Geometry: final body of the model. Coordinates: model frame, mm. A direction names the side the tool comes from. Coordinates: 2 decimals unless noted, no trailing zeros. Order: outer loops, then holes, each group sorted by start corner. A loop starts at its lowest first (then second) coordinate and runs counter-clockwise, first axis right, second up. Notation, with made-up numbers: M 12.5,32.25 L 46.5,32.25 A17 cw 46.5,62.25 Z; hole C -7,12 d4. An arc over 180 degrees is marked long. Write item = value, one per line. Start each with the question number.
```python
from build123d import *

# Parameters (mm, degrees)
F0_W     = 92.1045392752
F0_H     = 59.6973858774
F1_DEPTH = 25.4
F2_DEPTH = 25.4
F4_W     = 34.4229061157
F4_H     = 23.5688388348
F5_DEPTH = 70.612
F6_DEPTH = 99.568


with BuildPart() as f1:
    # F0 (on Front) → F1 (new body)
    with BuildSketch(Plane.XZ):
        with Locations((-26.6700014472, 29.8486929387)):
            Rectangle(F0_W, F0_H)
    extrude(amount=F1_DEPTH)

    # F2 (add): a face of the model
    f2_faces = [f1.faces().sort_by_distance(p)[0] for p in [
        (-26.6700014472, 0, 29.8486929387),
    ]]
    extrude(f2_faces, amount=F2_DEPTH)

    # F4 (on face) → F5 (cut)
    with BuildSketch(Plane.XZ.offset(25.4)):
        with Locations((-26.9801160321, 47.91296646)):
            Rectangle(F4_W, F4_H)
    extrude(amount=-F5_DEPTH, mode=Mode.SUBTRACT)

    # F3 (on face) → F6 (cut)
    with BuildSketch(Plane.YZ.offset(19.3822681904)):
        with BuildLine():
            Line((-25.4, 59.6973858774), (-25.4, 12.8698255867))
            ThreePointArc((-25.4, 12.8698255867), (1.6694190997, 29.9515872227), (13.4900575504, 59.6973858774))
            Line((13.4900575504, 59.6973858774), (-25.4, 59.6973858774))
        make_face()
    extrude(amount=-F6_DEPTH, mode=Mode.SUBTRACT)


solid = f1.part
```
Item 1: First-contact query: pin 1 (1.5 mm diameter, centred on x = -52, z = 28, fed in from -Y); pin 2 (6 mm diameter, centred on x = -24, y = 20, fed in from +Z). Flat tips, straight axial feed; report the tip coordinate or a pass-through.
Item 2: Material intervals for probe 1 along X at (y, z) = (18.5, 55.5); probe 2 along Y at (x, z) = (-64, 16); probe 3 along Z at (x, y) = (-11.5, 19), sorted ascending. Write a range as [from, to].
Item 3: Draft query along X for faces 1 (the flat face through (-9.769, 18, 48)), 2 (the flat face through (-44.192, 18, 48)), 3 (the flat face through (-72.722, 5, 23)), 4 (the flat face through (5, 19, 59.697)). Return one class per face: pulls with the +X half, pulls with the -X half, needs draft (parallel to the pull), parting line crosses it, or undercut.
Item 4: Section query A-A on y = 15. Output: boundary loops of the cut face in (x, z).
Item 5: Section query C-C on x = -5. Output: boundary loops of the cut face in (y, z), and give its area (3 significant figures).
Item 6: Reachability of faces 5 (the flat face through (19.382, 5, 23)), 6 (the flat face through (-27, 16, 36.129)) from +Z, -Z, +X, -X, +Y, -Y: full face, straight path, thin tool, end or side. Return the list, or none.
Item 7: Section query D-D on z = 46. Output: boundary loops of the cut face in (x, y).
Item 8: Section query B-B on z = 56.5. Output: boundary loops of the cut face in (x, y), and give its area (3 significant figures).
Ans:
q1.pin_1 = -0.74
q1.pin_2 = 36.13
q2.probe_1 = [-72.72, -44.19], [-9.77, 19.38]
q2.probe_2 = [-16.53, 25.4]
q2.probe_3 = [0, 36.13]
q3.face_1 = undercut
q3.face_2 = undercut
q3.face_3 = pulls with the -X half
q3.face_4 = needs draft
q4.outline = M -72.72,0 L 19.38,0 L 19.38,59.7 L -9.77,59.7 L -9.77,36.13 L -44.19,36.13 L -44.19,59.7 L -72.72,59.7 Z
q5.outline = M -25.4,0 L 25.4,0 L 25.4,59.7 L 13.49,59.7 A51.69 cw -25.4,12.87 Z
q5.area = 1,710 mm^2
q6.face_5 = +Z, -Z, +X, +Y, -Y
q6.face_6 = +Z, +Y, -Y
q7.outline = M -72.72,10.73 L -44.19,10.73 L -44.19,25.4 L -72.72,25.4 Z; M -9.77,10.73 L 19.38,10.73 L 19.38,25.4 L -9.77,25.4 Z
q8.outline = M -72.72,13.19 L -44.19,13.19 L -44.19,25.4 L -72.72,25.4 Z; M -9.77,13.19 L 19.38,13.19 L 19.38,25.4 L -9.77,25.4 Z
q8.area = 704 mm^2
